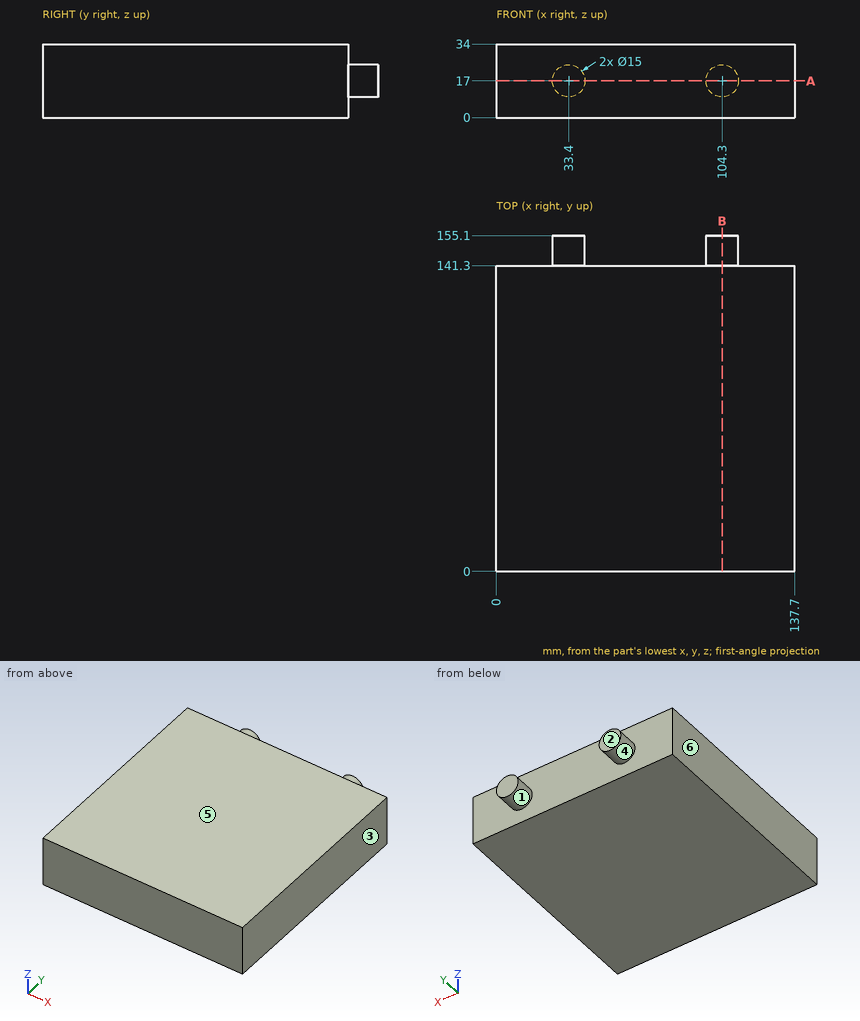
Input: dimensioned drawing with shaded views. Units: mm. Origin: part minimum x, y, z. A direction names the side the tool comes from. Round coordinates to 2 decimals unless told otherwise and drop trailing zeros. Order: outer loops, then holes, each group sorted by start corner. A loop starts at its lowest first (then second) coordinate and runs counter-clockwise, first axis right, second up. Notation, with made-up numbers: (-37, 36.5) -> (-31, 36.5) arc R28 ccw to (-31, 68.5) -> close; hole circle Ø1 at (-0.75, 37). An arc over 180 degrees is marked (long way). One line per item, written item: value. Start each with the question number.
Q1. Pin query (flat end, axial travel): pin 1 (3 mm diameter, centred on x = 97, z = 12, fed in from -Y); pin 2 (2 mm diameter, centred on x = 98.5, z = 28, fed in from +Y). Return the tip coordinate at first contact, or that it passes through.
Q2. Draft query along X for the marked faces 3, 4, 5 and 6. Return one class per face: pulls with the +X half, pulls with the -X half, needs draft (parallel to the pull), parting line crosses it, or undercut.
Q3. Section query A-A (z = 17). Return the cut outline in (x, y), plus the area to 3 significant figures.
Q4. Material intervals for probe 1 along Y at (x, z) = (96.5, 23); probe 2 along X at (y, z) = (148.5, 22), sorted ascending.
Q5. Access query for the marked faces 1 and 2. Directions: +Z, -Z, +X, -X, +Y, -Y. A direction counts if a zero-diameter tool reaches every point of the face in a straight line with its end or side. Return the directions, or none.
Q6. Section query B-B (x = 104.3). Return the cut outline in (y, z).
Findings below:
1. pin 1: y = 0
1. pin 2: y = 141.3
2. face 3: pulls with the +X half
2. face 4: undercut
2. face 5: needs draft
2. face 6: pulls with the -X half
3. outline: (0, 0) -> (137.7, 0) -> (137.7, 141.3) -> (111.8, 141.3) -> (111.8, 155.1) -> (96.8, 155.1) -> (96.8, 141.3) -> (40.9, 141.3) -> (40.9, 155.1) -> (25.9, 155.1) -> (25.9, 141.3) -> (0, 141.3) -> close
3. area: 19,900 mm²
4. probe 1: 0 to 141.3
4. probe 2: 27.81 to 38.99, 98.71 to 109.89
5. face 1: +Y
5. face 2: +Z, -Z, +X, -X, +Y
6. outline: (0, 0) -> (141.3, 0) -> (141.3, 9.5) -> (155.1, 9.5) -> (155.1, 24.5) -> (141.3, 24.5) -> (141.3, 34) -> (0, 34) -> close
